Source: CAD feature listing. Evaluate the final solid. Frame: model axes, mm. Give positions to 0.01 mm unless a question says otherwise; leave off trailing zeros. Order: outer loops, then holes, each group sorted by start corner. A loop starts at its lowest first (then second) coordinate and runs counter-clockwise, first axis right, second up.
```python
from build123d import *

# Parameters (mm, degrees)
SKETCH1_W           = 30
SKETCH1_H           = 3
BOSS_EXTRUDE1_DEPTH = 3


with BuildPart() as part:
    # Sketch1 → Boss-Extrude1 (new body)
    with BuildSketch(Plane(origin=(0, 0, 0), x_dir=(1, 0, 0), z_dir=(0, 1, 0))):
        Polygon((0, 31), (0, 42), (203, 42), (203, 0), (0, 0), (0, 11), (3, 11), (3, 31), align=None)
        with Locations((48, 4.5)):
            Rectangle(SKETCH1_W, SKETCH1_H, mode=Mode.SUBTRACT)
        with Locations((158, 4.5)):
            Rectangle(SKETCH1_W, SKETCH1_H, mode=Mode.SUBTRACT)
        with Locations((158, 37.5)):
            Rectangle(SKETCH1_W, SKETCH1_H, mode=Mode.SUBTRACT)
        with Locations((48, 37.5)):
            Rectangle(SKETCH1_W, SKETCH1_H, mode=Mode.SUBTRACT)
    extrude(amount=BOSS_EXTRUDE1_DEPTH)


solid = part.part
```
1) Material intervals for L1, parallel to Z at x = 55.5, y = 1.55; L2, parallel to X at y = 1.55, z = -5; L3, parallel to X at y = 2.7, z = -16, sorted ascending.
Report:
L1: z = -42 to -39, -36 to -6, -3 to 0
L2: x = 0 to 33, 63 to 143, 173 to 203
L3: x = 3 to 203
2) Section query B-B, the plane y = 0.55. Return the cut outline in (x, z).
Report:
outline: (0, -42) - (203, -42) - (203, 0) - (0, 0) - (0, -11) - (3, -11) - (3, -31) - (0, -31) - close; hole (33, -39) - (63, -39) - (63, -36) - (33, -36) - close; hole (33, -6) - (63, -6) - (63, -3) - (33, -3) - close; hole (143, -39) - (173, -39) - (173, -36) - (143, -36) - close; hole (143, -6) - (173, -6) - (173, -3) - (143, -3) - close
3) Pin query (flat end, axial travel): pin 1 (1 mm diameter, centred on y = 0.5, z = -13.5, fed in from -X). Return the tip coordinate at first contact, or that it passes through.
Report:
pin 1: stops at x = 3
4) Section query A-A, the plane x = 58.5. Return the cut outline in (y, z), and give its area (3 significant figures).
Report:
outline: (0, -42) - (3, -42) - (3, -39) - (0, -39) - close; (0, -36) - (3, -36) - (3, -6) - (0, -6) - close; (0, -3) - (3, -3) - (3, 0) - (0, 0) - close
area: 108 mm2
